Source: CAD feature listing. Evaluate the final solid. Frame: model axes, mm. A direction names the side the tool comes from. Give positions to 0.01 mm unless a question says otherwise; leave off trailing zeros. Loops run counter-clockwise (first coordinate to the right, second up) from the corner with the lowest first, then second, coordinate; pieces in that order, holes last. Notation, with made-up numbers: M 5,-37.5 L 53,-37.5 A20 cw 53,0.5 Z; hole C -24.5,-18 d3. An arc over 180 degrees is marked long. Answer in a Markdown table with one row per item.
```python
from build123d import *

# Parameters (mm, degrees)
F1_DEPTH = 30
F2_R     = 4.4
F3_R     = 4.4
F4_DEPTH = 25
F5_R     = 2
F6_R     = 2


# Not quite as in the source:
# - a feature names something its author has since deleted; it is built from what else it names


with BuildPart() as f1:
    # F0 (on Front) → F1 (new body)
    with BuildSketch(Plane.XZ):
        Polygon((90, -1), (90, 1), (70, 1), (70, 99), (-70, 99), (-70, 1), (-90, 1), (-90, -1), (-68, -1), (-68, 97), (68, 97), (68, -1), align=None)
    extrude(amount=F1_DEPTH)

    # F2 (on face) + F3 (on face) → F4 (cut)
    with BuildSketch(Plane.XY.offset(1)):
        with Locations((-80, -15)):
            Circle(F2_R)
        with Locations((80, -15)):
            Circle(F2_R)
    with BuildSketch(Plane.XY.offset(99)):
        with Locations((-25, -15)):
            Circle(F3_R)
        with Locations((25, -15)):
            Circle(F3_R)
    extrude(amount=-F4_DEPTH, mode=Mode.SUBTRACT)

    # F5
    f5_edges = [f1.edges().sort_by_distance(p)[0] for p in [
        (-70, -15, 99),
        (70, -15, 99),
    ]]
    fillet(f5_edges, radius=F5_R)

    # F6
    f6_edges = [f1.edges().sort_by_distance(p)[0] for p in [
        (68, -15, -1),
        (-68, -15, -1),
    ]]
    fillet(f6_edges, radius=F6_R)


solid = f1.part
```
1) Section B-B, the plane x = -22.5. Return loops of the section in (y, z).
Reply:
| item | result |
|---|---|
| outline | M -30,97 L -18.62,97 L -18.62,99 L -30,99 Z; M -11.38,97 L 0,97 L 0,99 L -11.38,99 Z |
2) Pull-direction query (Y, two-part tool) for faces 1 (the flat face through (-1, -15, 97)), 2 (the flat face through (-0.4, -30, 97.4)), 3 (the cylindrical face through (27.365, -11.29, 98.014)); classes: released by +Y, released by -Y, zero draft, split by the parting line, or undercut.
Reply:
| item | result |
|---|---|
| face 1 | zero draft |
| face 2 | released by -Y |
| face 3 | undercut |
3) Material intervals for L1, parallel to X at y = -24.5, z = 43.5; L2, parallel to Y at x = 80, z = -0.4; L3, parallel to Z at x = -71.5, y = -26, sorted ascending.
Reply:
| item | result |
|---|---|
| L1 | x = -70 to -68, 68 to 70 |
| L2 | y = -30 to -19.4, -10.6 to 0 |
| L3 | z = -1 to 1 |
4) Section C-C, the plane y = -15. Count the separate pieces of the cut face and the enclosed holes in it, then the cut area to 3 significant figures.
Reply:
| item | result |
|---|---|
| separate pieces | 5 |
| enclosed holes | 0 |
| area | 678 mm² |
5) Pin query (flat end, axial travel): pin 1 Ø5 at (y, z) = (-8, 83.5) entering from -X; pin 2 Ø8 at (x, y) = (-80, -15) entering from +Z; pin 3 Ø2 at (x, y) = (51.5, -10.5) entering from -Z; pin 4 Ø10 at (x, y) = (77, -14.5) entering from +Z. Return the tip coordinate at first contact, or that it passes through.
Reply:
| item | result |
|---|---|
| pin 1 | stops at x = -70 |
| pin 2 | passes through |
| pin 3 | stops at z = 97 |
| pin 4 | stops at z = 1 |
6) Section A-A, the plane z = 34. Return loops of the section in (x, y), then the cut area to 3 significant figures.
Reply:
| item | result |
|---|---|
| outline | M -70,-30 L -68,-30 L -68,0 L -70,0 Z; M 68,-30 L 70,-30 L 70,0 L 68,0 Z |
| area | 120 mm² |
7) Set-up query: faces 4 (the flat face through (70, -15, 48)), 5 (the flat face through (-68, -15, 48)), 6 (the flat face through (-75, -15, 1)). Return all of +Z, -Z, +X, -X, +Y, -Y with unobstructed straight access to the full face (end or side cutting, diameter ignored); none if empty.
Reply:
| item | result |
|---|---|
| face 4 | +Z, +X, +Y, -Y |
| face 5 | -Z, +Y, -Y |
| face 6 | +Z, -X, +Y, -Y |
8) Section D-D, the plane y = -6.5. Return loops of the section in (x, z).
Reply:
| item | result |
|---|---|
| outline | M -90,-1 L -70,-1 A2 ccw -68,1 L -68,97 L 68,97 L 68,1 A2 ccw 70,-1 L 90,-1 L 90,1 L 70,1 L 70,97 A2 ccw 68,99 L -68,99 A2 ccw -70,97 L -70,1 L -90,1 Z |
